from build123d import *

# Parameters (mm, degrees)
BOSS_EXTRUDE1_DEPTH              = 4.7625
BOSS_EXTRUDE1_DEPTH_BACK         = 4.7625
SKETCH3_W                        = 382.27
SKETCH3_H                        = 38.1
FILLET1_R                        = 0.314325
TAP_DRILL_FOR_10_32_TAP1_D       = 4.0386
TAP_DRILL_FOR_10_32_TAP1_DEPTH   = 25.4
TAP_DRILL_FOR_10_32_TAP1_TIP     = 1.213317848
TAP_DRILL_FOR_10_32_TAP2_D       = 4.0386
TAP_DRILL_FOR_10_32_TAP2_DEPTH   = 25.4
TAP_DRILL_FOR_10_32_TAP2_TIP     = 1.213317848
SKETCH10_W                       = 19.05
SKETCH10_H                       = 2.286
CUT_EXTRUDE1_DEPTH               = 195.953531979
F_10_CLEARANCE_HOLE1_D           = 4.9784
F_10_CLEARANCE_HOLE1_CSINK_D     = 10.4394
F_10_CLEARANCE_HOLE1_CSINK_ANGLE = 82
CUT_EXTRUDE2_DEPTH               = 2.54
F_10_CLEARANCE_HOLE2_D           = 4.9784


with BuildPart() as part:
    # Sketch3 → Boss-Extrude1 (new, two sides: drawn at the far end of the back side and taken through both)
    with BuildSketch(Plane(origin=(0, 0, 0), x_dir=(1, 0, 0), z_dir=(0, 1, 0)).offset(-BOSS_EXTRUDE1_DEPTH_BACK)):
        Rectangle(SKETCH3_W, SKETCH3_H)
    extrude(amount=BOSS_EXTRUDE1_DEPTH + BOSS_EXTRUDE1_DEPTH_BACK)

    # Fillet1
    fillet1_edges = [part.edges().sort_by_distance(p)[0] for p in [
        (0, 4.7625, 19.05),
        (0, -4.7625, -19.05),
        (0, 4.7625, -19.05),
        (0, -4.7625, 19.05),
    ]]
    fillet(fillet1_edges, radius=FILLET1_R)

    # Tap Drill for #10-32 Tap1
    with Locations(Plane.ZY.offset(191.135)):
        with Locations((-13.97, -0.762), (13.97, -0.762)):
            Hole(TAP_DRILL_FOR_10_32_TAP1_D / 2, depth=TAP_DRILL_FOR_10_32_TAP1_DEPTH)
            with Locations((0, 0, -(TAP_DRILL_FOR_10_32_TAP1_DEPTH + TAP_DRILL_FOR_10_32_TAP1_TIP / 2))):  # 118° drill point
                Cone(0, TAP_DRILL_FOR_10_32_TAP1_D / 2, TAP_DRILL_FOR_10_32_TAP1_TIP, mode=Mode.SUBTRACT)

    # Tap Drill for #10-32 Tap2
    with Locations(Plane(origin=(191.135, 0, 0), x_dir=(0, 0, -1), z_dir=(1, 0, 0))):
        with Locations((-13.97, -0.762), (13.97, -0.762)):
            Hole(TAP_DRILL_FOR_10_32_TAP2_D / 2, depth=TAP_DRILL_FOR_10_32_TAP2_DEPTH)
            with Locations((0, 0, -(TAP_DRILL_FOR_10_32_TAP2_DEPTH + TAP_DRILL_FOR_10_32_TAP2_TIP / 2))):  # 118° drill point
                Cone(0, TAP_DRILL_FOR_10_32_TAP2_D / 2, TAP_DRILL_FOR_10_32_TAP2_TIP, mode=Mode.SUBTRACT)

    # Sketch10 → Cut-Extrude1 (cut, through all)
    with BuildSketch(Plane(origin=(0, 0, -19.05), x_dir=(-1, 0, 0), z_dir=(0, 0, -1))):
        with BuildLine():
            Line((159.385, 4.7625), (159.385, 3.175))
            ThreePointArc((159.385, 3.175), (158.45506403, 0.92993597), (156.21, 0))
            Line((156.21, 0), (-99.06, 0))
            ThreePointArc((-99.06, 0), (-101.30506403, 0.92993597), (-102.235, 3.175))
            Line((-102.235, 3.175), (-102.235, 4.7625))
            Line((-102.235, 4.7625), (159.385, 4.7625))
        make_face()
        with Locations((-181.61, 3.6195)):
            Rectangle(SKETCH10_W, SKETCH10_H)
    extrude(amount=-CUT_EXTRUDE1_DEPTH, mode=Mode.SUBTRACT)

    # #10 Clearance Hole1 (through all)
    with Locations(Plane(origin=(0, -4.7625, 0), x_dir=(-1, 0, 0), z_dir=(0, -1, 0))):
        with Locations((-114.935, 12.7), (-146.685, 12.7), (-146.685, -12.7), (-114.935, -12.7)):
            CounterSinkHole(F_10_CLEARANCE_HOLE1_D / 2, F_10_CLEARANCE_HOLE1_CSINK_D / 2, counter_sink_angle=F_10_CLEARANCE_HOLE1_CSINK_ANGLE)

    # Sketch17 → Cut-Extrude2 (cut)
    with BuildSketch(Plane(origin=(0, 2.4765, 0), x_dir=(1, 0, 0), z_dir=(0, 1, 0))):
        Polygon((191.135, 0), (191.135, 10.16), (172.085, 10.16), (172.085, -10.16), (191.135, -10.16), align=None)
    extrude(amount=-CUT_EXTRUDE2_DEPTH, mode=Mode.SUBTRACT)

    # #10 Clearance Hole2 (through all)
    with Locations(Plane(origin=(0, 0, 0), x_dir=(1, 0, 0), z_dir=(0, 1, 0))):
        with Locations((-141.418780002, 12.7), (-141.418780002, -12.7), (17.331219998, 12.7), (17.331219998, -12.7)):
            Hole(F_10_CLEARANCE_HOLE2_D / 2)


solid = part.part
CAD build for the part. Positions are in the model's coordinates, mm. A direction names the side the tool comes from. Give positions to 0.01 mm unless a question says otherwise; leave off trailing zeros. Write each loop counter-clockwise with the first axis right and the second up, starting at its lowest first coordinate (ties: lowest second). Pieces come first, ordered by that corner, then holes. Notation, with made-up numbers: (29.5, 38) -> (74.5, 38) arc R31 ccw to (74.5, 67) -> close; hole circle Ø2 at (-15, -24). An arc over 180 degrees is marked (long way). Return JSON: item names as keys, results as strings.
Item 1: Drop flat-ended pins along their axis: pin 1 (6.5 mm diameter, centred on x = 114.935, z = 12.7, fed in from -Y); pin 2 (3 mm diameter, centred on y = -0.762, z = 13.97, fed in from +X); pin 3 (4.5 mm diameter, centred on x = 181, z = -16, fed in from +Y); pin 4 (8 mm diameter, centred on x = 146.685, z = 12.7, fed in from +Y). Give the stop position or say it passes through.
Answer below:
{"pin 1": "stops at y = -2.5", "pin 2": "stops at x = 165.42", "pin 3": "stops at y = 2.48", "pin 4": "stops at y = 4.76"}
Item 2: Band-saw the part on B-B (x = 70). List the corners of the cut face in (y, z), then the cut area to 3 significant figures.
Answer below:
{"outline": "(-4.76, -18.74) arc R0.31 ccw to (-4.45, -19.05) -> (0, -19.05) -> (0, 19.05) -> (-4.45, 19.05) arc R0.31 ccw to (-4.76, 18.74) -> close", "area": "181 mm2"}
Item 3: Tool access for faces 1 (the flat face through (-30, 0, 0)), 2 (the flat face through (181, -0.063, 0)), 3 (the flat face through (182, 2.476, 15)): list every direction of +Z, -Z, +X, -X, +Y, -Y with a clear straight run to the whole face (end or side of a thin tool).
Answer below:
{"face 1": "+Z, -Z, +Y", "face 2": "+X, +Y", "face 3": "+Z, -Z, +X, +Y"}
Item 4: Drill centre lines: probe 1 along Z at (x, y) = (-170.5, -0.5); probe 2 along X at (y, z) = (-3, 11.5) (3 decimals); probe 3 along X at (y, z) = (-1.1, -12.7). Where is each one in solid material? Low to high.
Answer below:
{"probe 1": "z = -19.05 to -15.97, -11.97 to 11.97, 15.97 to 19.05", "probe 2": "x = -191.135 to -143.6, -139.238 to 15.15, 19.512 to 111.448, 118.422 to 143.198, 150.172 to 191.135", "probe 3": "x = -165.31 to -143.91, -138.93 to 14.84, 19.82 to 112.45, 117.42 to 144.2, 149.17 to 165.31"}
Item 5: Two-plate mould, pull along X, no slides. Class faces 4 (the flat face through (191.135, -2, 0)), 5 (the flat face through (-191.135, 0, 0)), 6 (the conical face through (117.436, -1.774, -13.488)), 7 (the flat face through (-175, 4.762, 0)): +X half, -X half, draft (parallel to the pull), parting line (faces both ways), or undercut.
Answer below:
{"face 4": "+X half", "face 5": "-X half", "face 6": "undercut", "face 7": "draft"}
